Could you check a few things on this model? Use its own coordinates, in mm. Face numbers are marked on the shaded views. Give positions to 0.01 mm unless a question says otherwise; leave off trailing zeros. Loops run counter-clockwise (first coordinate to the right, second up) from the corner with the lowest first, then second, coordinate; pieces in that order, holes last.
1. I need wall thicknesses on line 1 along Z through (x, y) = (-0.25, 10); line 2 along Z through (x, y) = (-0.25, 10.75); line 3 along X through (y, z) = (4, 0). Which ranges of each line are inside material? Lowest first, please.
2. Imagine slicing it at B-B (y = 4.25). List the corners of the cut face in (x, z) for me.
3. Thinking about a two-plate mould opening in Z: for the marked faces 1, 2 and 3, which applies, +Z half, -Z half, draft (parallel to the pull), parting line (faces both ways), or undercut?
4. For P1, Ø3, axis at x = 0.5, z = -0.5, coming from the +Y side; P2, Ø2, axis at x = 1.5, y = 5.5, coming from the -Z side; P3, Ø2, axis at x = 2, z = -1.5, coming from the -Y side; P4, Ø3, axis at x = -1, z = 1.5, coming from the +Y side, each with a flat end and sliding along its axis, tell me the tip position at first contact or that it passes through.
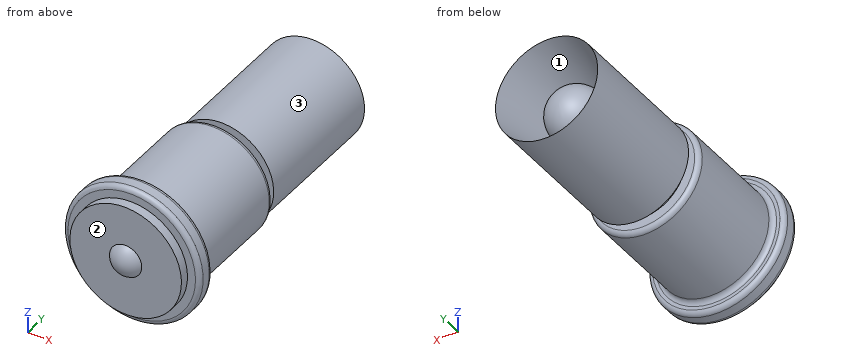
```python
from build123d import *

# Parameters (mm, degrees)
SKETCH2_W = 3
SKETCH2_H = 0.5
FILLET1_R = 0.25


with BuildPart() as part:
    # Sketch1 → Revolve1 (revolve)
    with BuildSketch(Plane(origin=(0, 0, 0), x_dir=(0, 0, -1), z_dir=(1, 0, 0)), mode=Mode.PRIVATE) as revolve1_sk:
        Polygon((0, 0), (3.68, 0), (3.68, 1), (3, 1), (3, 7), (2.25, 7), (2.25, 7.5), (2.75, 7.5), (2.75, 15), (0, 15), align=None)
    revolve(revolve1_sk.sketch.rotate(Axis((0, 15, 0), (0, -1, 0)), 180), axis=Axis((0, 15, 0), (0, -1, 0)))

    # Sketch2 → Revolve2 (revolve)
    with BuildSketch(Plane(origin=(0, 0, 0), x_dir=(0, 0, -1), z_dir=(1, 0, 0)), mode=Mode.PRIVATE) as revolve2_sk:
        with Locations((1.5, -0.25)):
            Rectangle(SKETCH2_W, SKETCH2_H)
    revolve(revolve2_sk.sketch.rotate(Axis((0, 0, 0), (0, -1, 0)), 180), axis=Axis((0, 0, 0), (0, -1, 0)))

    # Sketch3 → Revolve3 (revolve)
    with BuildSketch(Plane(origin=(0, 0, 0), x_dir=(0, 0, -1), z_dir=(1, 0, 0))):
        with BuildLine():
            Line((0, -1), (0, 1))
            ThreePointArc((0, 1), (1, 0), (0, -1))
        make_face()
    revolve(axis=Axis((0, -1, 0), (0, 1, 0)))

    # Fillet1
    fillet1_edges = [part.edges().sort_by_distance(p)[0] for p in [
        (0, 1, -3.68),
        (0, 0, -3.68),
        (0, 7, -3),
        (0, 1, -3),
    ]]
    fillet(fillet1_edges, radius=FILLET1_R)

    # Sketch5 → Cut-Revolve1 (revolve, cut)
    with BuildSketch(Plane(origin=(0, 0, 0), x_dir=(0, 0, -1), z_dir=(1, 0, 0))):
        Polygon((0, 15), (0, 8), (1.5, 8), (2.75, 15), align=None)
    revolve(axis=Axis((0, 15, 0), (0, -1, 0)), mode=Mode.SUBTRACT)

    # Sketch6 → Revolve4 (revolve)
    with BuildSketch(Plane(origin=(0, 0, 0), x_dir=(0, 0, -1), z_dir=(1, 0, 0))):
        with BuildLine():
            Line((0, 8), (0, 12.5))
            Line((0, 12.5), (0, 14))
            ThreePointArc((0, 14), (1.060660172, 13.560660172), (1.5, 12.5))
            Line((1.5, 12.5), (1.5, 8))
            Line((1.5, 8), (0, 8))
        make_face()
    revolve(axis=Axis((0, 8, 0), (0, 1, 0)))


solid = part.part
```
Derived:
1. line 1: z = -2.74 to -1.84, -1.48 to 1.48, 1.84 to 2.74
1. line 2: z = -2.74 to -1.98, -1.48 to 1.48, 1.98 to 2.74
1. line 3: x = -3 to 3
2. outline: circle Ø6 at (0, 0)
3. face 1: undercut
3. face 2: draft
3. face 3: parting line
4. P1: stops at y = 14
4. P2: stops at z = -2.96
4. P3: stops at y = -0.5
4. P4: stops at y = 15
